Could you check a few things on this drawing? It's one solid part, dimensions in mm from its lowest x, y, z. A direction names the side the tool comes from. Coordinates: 2 decimals unless noted, no trailing zeros. Order: outer loops, then holes, each group sorted by start corner. A loop starts at its lowest first (then second) coordinate and runs counter-clockwise, first axis right, second up.
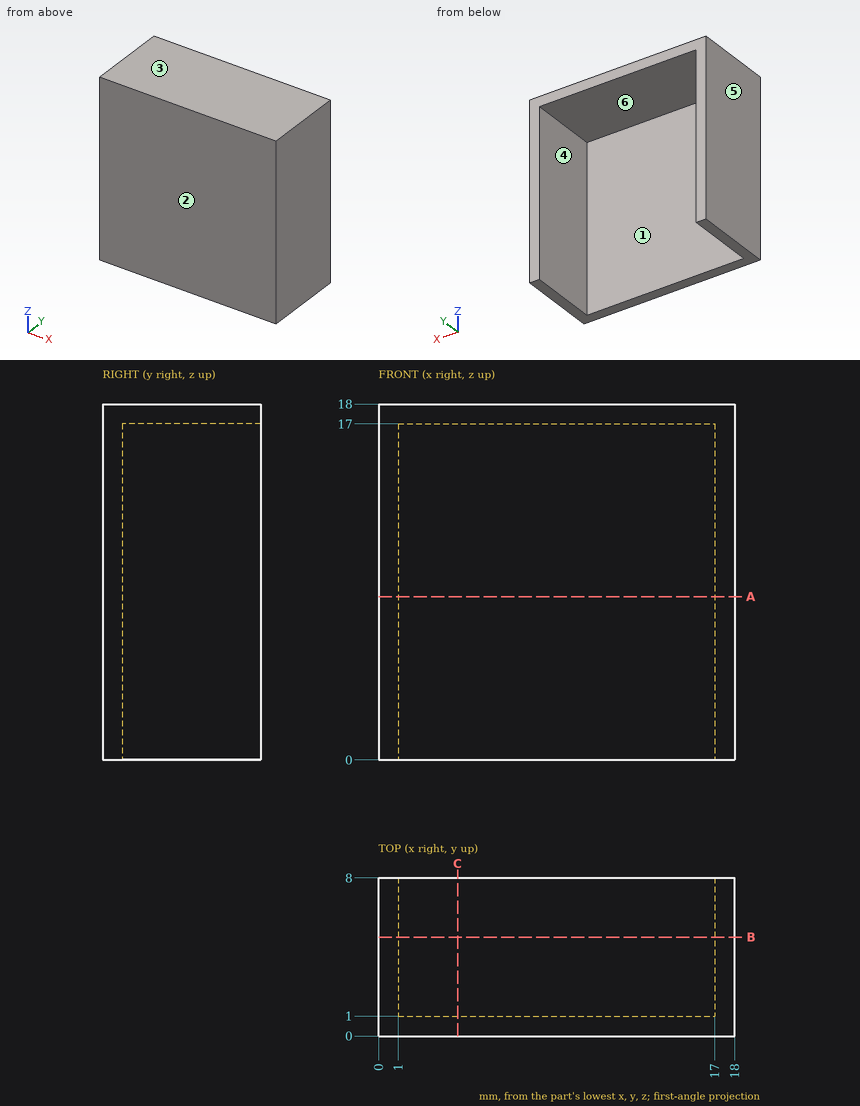
Item 1: Suppose I cut it at C-C (x = 4). List the corners of the cut face in (y, z) for me, and give its area (3 significant figures).
Item 2: For pin 1 Ø3 at (x, y) = (12, 3) entering from -Z; pin 2 Ø4 at (x, z) = (9.5, 10) entering from +Y, each with a flat end and sliding along its axis, tell me the tip position at first contact or that it passes through.
Item 3: Suppose I cut it at A-A (z = 8.25). List the corners of the cut face in (x, y) for me, and give its area (3 significant figures).
Item 4: Suppose I cut it at B-B (y = 5). List the corners of the cut face in (x, z) for me, and give its area (3 significant figures).
Item 5: Which directions (+Z, -Z, +X, -X, +Y, -Y) give clear straight access to the entire face, cutting with the end or side of a thin tool? Please do the marked faces 1 and 2.
Item 6: Thinking about a two-plate mould opening in X: for the marked faces 3, 4, 5 and 6, which applies, +X half, -X half, draft (parallel to the pull), parting line (faces both ways), or undercut?
Item 7: I need wall thicknesses on line 1 (X direction, y = 4.5, z = 7.75); line 2 (Z direction, x = 1.5, y = 1.75); line 3 (Y direction, x = 8.25, z = 15.25). Which ranges of each line are inside material? Lowest first, please.
Geometry results:
1. outline: (0, 0) - (1, 0) - (1, 17) - (8, 17) - (8, 18) - (0, 18) - close
1. area: 25.0 mm2
2. pin 1: stops at z = 17
2. pin 2: stops at y = 1
3. outline: (0, 0) - (18, 0) - (18, 8) - (17, 8) - (17, 1) - (1, 1) - (1, 8) - (0, 8) - close
3. area: 32.0 mm2
4. outline: (0, 0) - (1, 0) - (1, 17) - (17, 17) - (17, 0) - (18, 0) - (18, 18) - (0, 18) - close
4. area: 52.0 mm2
5. face 1: -Z, +Y
5. face 2: +Z, -Z, +X, -X, -Y
6. face 3: draft
6. face 4: undercut
6. face 5: -X half
6. face 6: undercut
7. line 1: x = 0 to 1, 17 to 18
7. line 2: z = 17 to 18
7. line 3: y = 0 to 1
